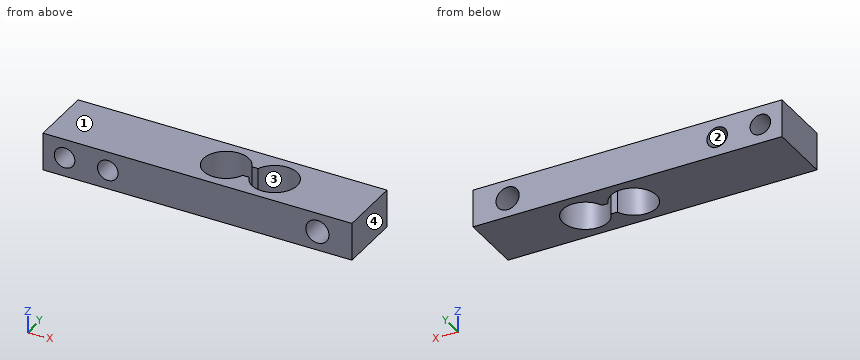
from build123d import *

# Parameters (mm, degrees)
SKETCH1_W               = 57.2
SKETCH1_H               = 11.7
BOSS_EXTRUDE1_DEPTH     = 7
CUT_EXTRUDE1_DEPTH      = 59.802465935
CUT_EXTRUDE1_DEPTH_BACK = 59.802465935
SKETCH2_R               = 2.15
SKETCH2_R_2             = 1.9
CUT_EXTRUDE2_DEPTH      = 59.802465935


with BuildPart() as part:
    # Sketch1 → Boss-Extrude1 (new body)
    with BuildSketch(Plane.XY):
        with Locations((28.6, 5.85)):
            Rectangle(SKETCH1_W, SKETCH1_H)
    extrude(amount=BOSS_EXTRUDE1_DEPTH)

    # Sketch2 → Cut-Extrude1 (cut, two sides: drawn at the far end of the back side and taken through both)
    with BuildSketch(Plane(origin=(0, 11.7, 0), x_dir=(1, 0, 0), z_dir=(0, 1, 0)).offset(-CUT_EXTRUDE1_DEPTH_BACK)):
        with Locations(Location((50.8, -3.5, 0), (0, 0, 270))):
            Circle(SKETCH2_R)
        with Locations(Location((4, -3.5, 0), (0, 0, 270))):
            Circle(SKETCH2_R_2)
        with Locations(Location((12, -3.5, 0), (0, 0, 270))):
            Circle(SKETCH2_R_2)
    extrude(amount=CUT_EXTRUDE1_DEPTH + CUT_EXTRUDE1_DEPTH_BACK, mode=Mode.SUBTRACT)

    # Sketch3 → Cut-Extrude2 (cut, through all)
    with BuildSketch(Plane.XY.offset(7)):
        with BuildLine():
            Line((34.57071198, 7.367429549), (35.734206681, 7.367429549))
            ThreePointArc((35.734206681, 7.367429549), (43.82348168, 5.85), (35.734206681, 4.332570451))
            Line((35.734206681, 4.332570451), (34.57071198, 4.332570451))
            ThreePointArc((34.57071198, 4.332570451), (26.48143698, 5.85), (34.57071198, 7.367429549))
        make_face()
    extrude(amount=-CUT_EXTRUDE2_DEPTH, mode=Mode.SUBTRACT)


solid = part.part
The listing builds one solid part. Answer for the finished solid, in the listing's coordinates (mm). Face numbers are marked on the shaded views. Coordinates: 2 decimals unless noted, no trailing zeros. Loops run counter-clockwise (first coordinate to the right, second up) from the corner with the lowest first, then second, coordinate; pieces in that order, holes last. Notation, with made-up numbers: M 31.5,-34 L 66.5,-34 A25 cw 66.5,-21 Z; hole C 9,-3.5 d7. An arc over 180 degrees is marked long. Answer in a Markdown table with one row per item.
1) Find section C-C (x = 50.8). Determine the outline of the cut face in (y, z), then the cut area to 3 significant figures.
Answers below:
| item | result |
|---|---|
| outline | M 0,0 L 11.7,0 L 11.7,1.35 L 0,1.35 Z; M 0,5.65 L 11.7,5.65 L 11.7,7 L 0,7 Z |
| area | 31.6 mm^2 |
2) Find section B-B (z = 3.5). Determine the outline of the cut face in (x, y).
Answers below:
| item | result |
|---|---|
| outline | M 0,0 L 2.1,0 L 2.1,11.7 L 0,11.7 Z; M 5.9,0 L 10.1,0 L 10.1,11.7 L 5.9,11.7 Z; M 13.9,0 L 48.65,0 L 48.65,11.7 L 13.9,11.7 Z; M 52.95,0 L 57.2,0 L 57.2,11.7 L 52.95,11.7 Z; hole M 34.57,4.33 L 35.73,4.33 A4.19 ccw long 35.73,7.37 L 34.57,7.37 A4.19 ccw long Z |
3) Find section A-A (y = 5.85). Determine the outline of the cut face in (x, z).
Answers below:
| item | result |
|---|---|
| outline | M 0,0 L 26.48,0 L 26.48,7 L 0,7 Z; M 43.82,0 L 57.2,0 L 57.2,7 L 43.82,7 Z; hole C 4,3.5 d3.8; hole C 12,3.5 d3.8; hole C 50.8,3.5 d4.3 |
4) Determine the mould class of the marked faces 1, 2, 3 and 4 for opening direction X: released by +X, released by -X, zero draft, split by the parting line, or undercut.
Answers below:
| item | result |
|---|---|
| face 1 | zero draft |
| face 2 | undercut |
| face 3 | undercut |
| face 4 | released by +X |
5) Find section D-D (y = 9). Determine the outline of the cut face in (x, z), then the cut area to 3 significant figures.
Answers below:
| item | result |
|---|---|
| outline | M 0,0 L 27.91,0 L 27.91,7 L 0,7 Z; M 33.43,0 L 36.88,0 L 36.88,7 L 33.43,7 Z; M 42.39,0 L 57.2,0 L 57.2,7 L 42.39,7 Z; hole C 4,3.5 d3.8; hole C 12,3.5 d3.8; hole C 50.8,3.5 d4.3 |
| area | 286 mm^2 |
6) Given pin 1 (0.9 mm diameter, centred on x = 35, z = 4, fed in from -Y); pin 2 (1 mm diameter, centred on x = 29, y = 8, fed in from +Z), each flat-ended and moving along its own axis, determine where each tip first touches the part or whether it passes through.
Answers below:
| item | result |
|---|---|
| pin 1 | y = 0 |
| pin 2 | through |
7) Find the intervals of material crossed by probe 1 along Z at (x, y) = (12, 6.25); probe 2 along X at (y, z) = (6.5, 3.5); probe 3 along X at (y, z) = (9, 1), in increasing order.
Answers below:
| item | result |
|---|---|
| probe 1 | 0 to 1.6, 5.4 to 7 |
| probe 2 | 0 to 2.1, 5.9 to 10.1, 13.9 to 26.53, 43.77 to 48.65, 52.95 to 57.2 |
| probe 3 | 0 to 27.91, 33.43 to 36.88, 42.39 to 57.2 |
